```python
from build123d import *

# Parameters (mm, degrees)
SKETCH1_R           = 1.375
SKETCH1_R_2         = 6.25
BOSS_EXTRUDE1_DEPTH = 3


with BuildPart() as part:
    # Sketch1 → Boss-Extrude1 (new body)
    with BuildSketch(Plane.XY):
        with BuildLine():
            Line((-75, 23), (-75, -23))
            Line((-75, -23), (-55.658312395, -23))
            ThreePointArc((-55.658312395, -23), (-54.792286991, -23.127718677), (-54, -23.5))
            ThreePointArc((-54, -23.5), (-50, -27.5), (-46, -23.5))
            ThreePointArc((-46, -23.5), (-45.207713009, -23.127718677), (-44.341687605, -23))
            Line((-44.341687605, -23), (-25.658312395, -23))
            ThreePointArc((-25.658312395, -23), (-24.792286991, -23.127718677), (-24, -23.5))
            ThreePointArc((-24, -23.5), (-20, -27.5), (-16, -23.5))
            ThreePointArc((-16, -23.5), (-15.207713009, -23.127718677), (-14.341687605, -23))
            Line((-14.341687605, -23), (14.341687605, -23))
            ThreePointArc((14.341687605, -23), (15.207713009, -23.127718677), (16, -23.5))
            ThreePointArc((16, -23.5), (20, -27.5), (24, -23.5))
            ThreePointArc((24, -23.5), (24.792286991, -23.127718677), (25.658312395, -23))
            Line((25.658312395, -23), (44.341687605, -23))
            ThreePointArc((44.341687605, -23), (45.207713009, -23.127718677), (46, -23.5))
            ThreePointArc((46, -23.5), (50, -27.5), (54, -23.5))
            ThreePointArc((54, -23.5), (54.792286991, -23.127718677), (55.658312395, -23))
            Line((55.658312395, -23), (75, -23))
            Line((75, -23), (75, 23))
            Line((75, 23), (55.658312395, 23))
            ThreePointArc((55.658312395, 23), (54.792286991, 23.127718677), (54, 23.5))
            ThreePointArc((54, 23.5), (50, 27.5), (46, 23.5))
            ThreePointArc((46, 23.5), (45.207713009, 23.127718677), (44.341687605, 23))
            Line((44.341687605, 23), (25.658312395, 23))
            ThreePointArc((25.658312395, 23), (24.792286991, 23.127718677), (24, 23.5))
            ThreePointArc((24, 23.5), (20, 27.5), (16, 23.5))
            ThreePointArc((16, 23.5), (15.207713009, 23.127718677), (14.341687605, 23))
            Line((14.341687605, 23), (-14.341687605, 23))
            ThreePointArc((-14.341687605, 23), (-15.207713009, 23.127718677), (-16, 23.5))
            ThreePointArc((-16, 23.5), (-20, 27.5), (-24, 23.5))
            ThreePointArc((-24, 23.5), (-24.792286991, 23.127718677), (-25.658312395, 23))
            Line((-25.658312395, 23), (-44.341687605, 23))
            ThreePointArc((-44.341687605, 23), (-45.207713009, 23.127718677), (-46, 23.5))
            ThreePointArc((-46, 23.5), (-50, 27.5), (-54, 23.5))
            ThreePointArc((-54, 23.5), (-54.792286991, 23.127718677), (-55.658312395, 23))
            Line((-55.658312395, 23), (-75, 23))
        make_face()
        with Locations((-50, -23.5)):
            Circle(SKETCH1_R, mode=Mode.SUBTRACT)
        with Locations((-20, -23.5)):
            Circle(SKETCH1_R, mode=Mode.SUBTRACT)
        with Locations((20, -23.5)):
            Circle(SKETCH1_R, mode=Mode.SUBTRACT)
        with Locations((50, -23.5)):
            Circle(SKETCH1_R, mode=Mode.SUBTRACT)
        with Locations((50, 23.5)):
            Circle(SKETCH1_R, mode=Mode.SUBTRACT)
        with Locations((20, 23.5)):
            Circle(SKETCH1_R, mode=Mode.SUBTRACT)
        with Locations((-20, 23.5)):
            Circle(SKETCH1_R, mode=Mode.SUBTRACT)
        with Locations((-50, 23.5)):
            Circle(SKETCH1_R, mode=Mode.SUBTRACT)
        with Locations((-55.192693601, 8)):
            Circle(SKETCH1_R_2, mode=Mode.SUBTRACT)
        with Locations((-23.192693601, 8)):
            Circle(SKETCH1_R_2, mode=Mode.SUBTRACT)
        with Locations((8.807306399, 8)):
            Circle(SKETCH1_R_2, mode=Mode.SUBTRACT)
        with Locations((40.807306399, 8)):
            Circle(SKETCH1_R_2, mode=Mode.SUBTRACT)
        with Locations((-39.192693601, -8)):
            Circle(SKETCH1_R_2, mode=Mode.SUBTRACT)
        with Locations((-7.192693601, -8)):
            Circle(SKETCH1_R_2, mode=Mode.SUBTRACT)
        with Locations((24.807306399, -8)):
            Circle(SKETCH1_R_2, mode=Mode.SUBTRACT)
        with Locations((56.807306399, -8)):
            Circle(SKETCH1_R_2, mode=Mode.SUBTRACT)
    extrude(amount=BOSS_EXTRUDE1_DEPTH)


solid = part.part
```
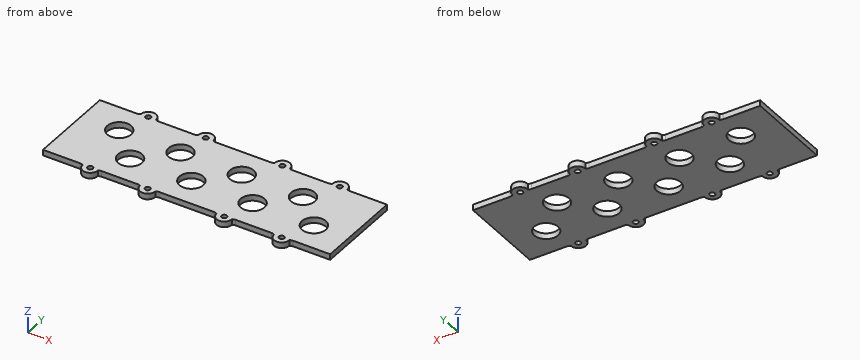
Check sheet for the modelled part. Datum: model origin and axes. Units: mm. Give positions to 0.01 mm unless a question says otherwise; leave off trailing zeros. Loops run counter-clockwise (first coordinate to the right, second up) from the corner with the lowest first, then second, coordinate; pieces in that order, holes last. Notation, with made-up numbers: M 70.5,-24.75 L 102.5,-24.75 A19 ccw 102.5,-0.75 Z; hole C 64.25,7 d2. An arc over 180 degrees is marked long. Answer as CSV lines item,"result".
Item 1: Scan lines: L1, parallel to X at y = 7.5, z = 2.7; L2, parallel to X at y = -13.5, z = 1.2; L3, parallel to Y at x = -50, z = 2.35 (3 decimals). Record each from-to range of solid material in increasing order.
Reply:
L1,"-75 to -61.42, -48.96 to -29.42, -16.96 to 2.58, 15.04 to 34.58, 47.04 to 75"
L2,"-75 to -42.16, -36.22 to -10.16, -4.22 to 21.84, 27.78 to 53.84, 59.78 to 75"
L3,"-27.5 to -24.875, -22.125 to 4.522, 11.478 to 22.125, 24.875 to 27.5"
Item 2: Sectioned sample at C-C, the plane x = 41. Enter the section's corners in (y, z), then the cut area to 3 significant figures.
Reply:
outline,"M -23,0 L 1.75,0 L 1.75,3 L -23,3 Z; M 14.25,0 L 23,0 L 23,3 L 14.25,3 Z"
area,"101 mm^2"
Item 3: Sectioned sample at A-A, the plane y = -8. Enter the section's corners in (x, z), then the cut area to 3 significant figures.
Reply:
outline,"M -75,0 L -45.44,0 L -45.44,3 L -75,3 Z; M -32.94,0 L -13.44,0 L -13.44,3 L -32.94,3 Z; M -0.94,0 L 18.56,0 L 18.56,3 L -0.94,3 Z; M 31.06,0 L 50.56,0 L 50.56,3 L 31.06,3 Z; M 63.06,0 L 75,0 L 75,3 L 63.06,3 Z"
area,"300 mm^2"
Item 4: Sectioned sample at D-D, the plane z = 0.85. State how many separate pieces and enclosed holes the cut face has, then the cut area to 3 significant figures.
Reply:
separate pieces,"1"
enclosed holes,"16"
area,"6,110 mm^2"
Item 5: Sectioned sample at B-B, the plane x = -20. Enter the section's corners in (y, z) (3 decimals).
Reply:
outline,"M -27.5,0 L -24.875,0 L -24.875,3 L -27.5,3 Z; M -22.125,0 L 2.627,0 L 2.627,3 L -22.125,3 Z; M 13.373,0 L 22.125,0 L 22.125,3 L 13.373,3 Z; M 24.875,0 L 27.5,0 L 27.5,3 L 24.875,3 Z"
Item 6: Depth check by flat-ended pin: pin 1 Ø1 at (x, z) = (-52.5, 0.5) entering from +Y; pin 2 Ø0.9 at (x, z) = (39, 2) entering from +Y; pin 3 Ø0.9 at (x, z) = (0.5, 1.5) entering from -Y; pin 4 Ø1.6 at (x, y) = (50, 23.5) entering from +Z. Enter the tip coordinate at first touch or a pass-through.
Reply:
pin 1,"y = 26.96"
pin 2,"y = 23"
pin 3,"y = -23"
pin 4,"through"
